from build123d import *

# Parameters (mm, degrees)
SKETCH1_R           = 17.5
BOSS_EXTRUDE1_DEPTH = 3.175


with BuildPart() as part:
    # Sketch1 → Boss-Extrude1 (new body)
    with BuildSketch(Plane(origin=(0, 0, 0), x_dir=(0, 0, -1), z_dir=(1, 0, 0))):
        with BuildLine():
            Line((-299.628459553, 0), (-299.628459553, -35))
            Line((-299.628459553, -35), (-265.081967213, -35))
            ThreePointArc((-265.081967213, -35), (-265.124051275, -34.999527037), (-265.166134738, -34.999003472))
            Line((-265.166134738, -34.999003472), (269.561502977, -34.999003472))
            Line((269.561502977, -34.999003472), (269.561502977, 7.5))
            Line((269.561502977, 7.5), (269.561502977, 95))
            Line((269.561502977, 95), (-299.628459553, 95))
            Line((-299.628459553, 95), (-299.628459553, 0))
        make_face()
        with Locations((-264.709663373, 0)):
            Circle(SKETCH1_R, mode=Mode.SUBTRACT)
        with Locations((-164.709663373, 0)):
            Circle(SKETCH1_R, mode=Mode.SUBTRACT)
        with Locations((-64.709663373, 0)):
            Circle(SKETCH1_R, mode=Mode.SUBTRACT)
        with Locations((35.290336627, 0)):
            Circle(SKETCH1_R, mode=Mode.SUBTRACT)
        with Locations((135.290336627, 0)):
            Circle(SKETCH1_R, mode=Mode.SUBTRACT)
        with Locations((235.290336627, 0)):
            Circle(SKETCH1_R, mode=Mode.SUBTRACT)
    extrude(amount=BOSS_EXTRUDE1_DEPTH)


solid = part.part
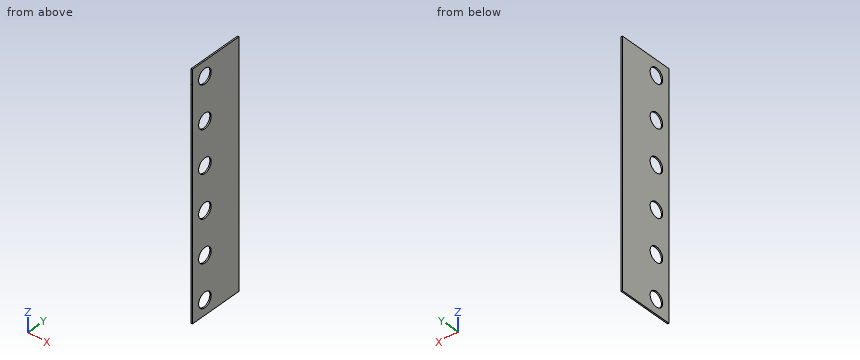
Check sheet for the modelled part. Datum: model origin and axes. Units: mm. Round coordinates to 2 decimals unless told otherwise and drop trailing zeros. Loops run counter-clockwise (first coordinate to the right, second up) from the corner with the lowest first, then second, coordinate; pieces in that order, holes last. Notation, with made-up numbers: M -39,16 L -20,16 A19 cw -20,26 Z; hole C -20,25 d3. An arc over 180 degrees is marked long. One line per question, with ' | ' between items. Start each with the question number.
Item 1: Section check B-B (y = 0). Record the boundary of the cut face in (x, z) (1 decimal), and give its area (3 significant figures).
Item 2: Section check A-A (x = 2.4). Record the boundary of the cut face in (y, z).
Item 3: Gauge pin test, flat end, axial feed: pin 1 Ø21 at (y, z) = (0, -235.29) entering from -X. Record the tip position at first contact, or that the pin passes through.
Item 4: Scan lines: probe 1 along Y at (x, z) = (2.35, -148); probe 2 along Y at (x, z) = (2.45, 156). Record each from-to range of solid material in increasing order.
Item 5: Section check C-C (z = -227.5). Record the boundary of the cut face in (x, y) (3 decimals).
Item 6: Section check D-D (z = -42). Record the boundary of the cut face in (x, y) (3 decimals), and give its area (3 significant figures).
Worked out:
1) outline: M 0,-269.6 L 3.2,-269.6 L 3.2,-252.8 L 0,-252.8 Z; M 0,-217.8 L 3.2,-217.8 L 3.2,-152.8 L 0,-152.8 Z; M 0,-117.8 L 3.2,-117.8 L 3.2,-52.8 L 0,-52.8 Z; M 0,-17.8 L 3.2,-17.8 L 3.2,47.2 L 0,47.2 Z; M 0,82.2 L 3.2,82.2 L 3.2,147.2 L 0,147.2 Z; M 0,182.2 L 3.2,182.2 L 3.2,247.2 L 0,247.2 Z; M 0,282.2 L 3.2,282.2 L 3.2,299.6 L 0,299.6 Z | area: 1,140 mm^2
2) outline: M -35,-269.56 L 95,-269.56 L 95,299.63 L -35,299.63 L -35,265.08 A35 cw -35,265.17 Z; hole C 0,-235.29 d35; hole C 0,-135.29 d35; hole C 0,-35.29 d35; hole C 0,64.71 d35; hole C 0,164.71 d35; hole C 0,264.71 d35
3) pin 1: through
4) probe 1: -35 to -12.03, 12.03 to 95 | probe 2: -35 to -15.18, 15.18 to 95
5) outline: M 0,-34.999 L 3.175,-34.999 L 3.175,-15.67 L 0,-15.67 Z; M 0,15.67 L 3.175,15.67 L 3.175,95 L 0,95 Z
6) outline: M 0,-34.999 L 3.175,-34.999 L 3.175,-16.163 L 0,-16.163 Z; M 0,16.163 L 3.175,16.163 L 3.175,95 L 0,95 Z | area: 310 mm^2
